from build123d import *

# Parameters (mm, degrees)
SKETCH1_W               = 28
SKETCH1_H               = 55
SKETCH1_R               = 1.25
BOSS_EXTRUDE1_DEPTH     = 6
SKETCH2_W               = 6
SKETCH2_H               = 55
BOSS_EXTRUDE2_DEPTH     = 14.5
SKETCH3_W               = 6
SKETCH3_H               = 55
BOSS_EXTRUDE3_DEPTH     = 48
SKETCH4_R               = 3
SKETCH4_R_2             = 11
CUT_EXTRUDE1_DEPTH      = 48
FILLET4_R               = 2
SKETCH5_W               = 21
SKETCH5_H               = 42
CUT_EXTRUDE2_DEPTH      = 10
FILLET5_R               = 2
ESQUISSE2_R             = 5
BOSS_EXTRU_3_DEPTH      = 41
ESQUISSE3_R             = 1.75
ENL_V_MAT_EXTRU_1_DEPTH = 105.928547117
ESQUISSE4_W             = 76
ESQUISSE4_H             = 20.5
BOSS_EXTRU_4_DEPTH      = 14
ESQUISSE5_W             = 76
ESQUISSE5_H             = 20.5
BOSS_EXTRU_5_DEPTH      = 14
ESQUISSE7_R             = 5
BOSS_EXTRU_8_DEPTH      = 26.5
ESQUISSE10_R            = 1.75
ENL_V_MAT_EXTRU_2_DEPTH = 113.898184219
ENL_V_MAT_EXTRU_3_DEPTH = 4.1
ENL_V_MAT_EXTRU_4_DEPTH = 4.1


with BuildPart() as part:
    # Sketch1 → Boss-Extrude1 (new body)
    with BuildSketch(Plane.XY):
        with Locations((14, 27.5)):
            Rectangle(SKETCH1_W, SKETCH1_H)
        with Locations((5, 52)):
            Circle(SKETCH1_R, mode=Mode.SUBTRACT)
        with Locations((15, 52)):
            Circle(SKETCH1_R, mode=Mode.SUBTRACT)
        with Locations((5, 3)):
            Circle(SKETCH1_R, mode=Mode.SUBTRACT)
        with Locations((15, 3)):
            Circle(SKETCH1_R, mode=Mode.SUBTRACT)
    extrude(amount=BOSS_EXTRUDE1_DEPTH)

    # Sketch2 → Boss-Extrude2 (add)
    with BuildSketch(Plane.XY.offset(6)):
        with Locations((25, 27.5)):
            Rectangle(SKETCH2_W, SKETCH2_H)
    extrude(amount=BOSS_EXTRUDE2_DEPTH)

    # Sketch3 → Boss-Extrude3 (add)
    with BuildSketch(Plane(origin=(28, 0, 0), x_dir=(0, 0, -1), z_dir=(1, 0, 0))):
        with Locations((-17.5, 27.5)):
            Rectangle(SKETCH3_W, SKETCH3_H)
    extrude(amount=BOSS_EXTRUDE3_DEPTH)

    # Sketch4 → Cut-Extrude1 (cut)
    with BuildSketch(Plane.XY.offset(20.5)):
        with Locations((61.416247904, 27.5)):
            Circle(SKETCH4_R)
        with Locations((34.041247904, 11.695036381)):
            Circle(SKETCH4_R)
        with Locations((34.041247904, 43.304963619)):
            Circle(SKETCH4_R)
        with Locations((43.166247904, 27.5)):
            Circle(SKETCH4_R_2)
    extrude(amount=-CUT_EXTRUDE1_DEPTH, mode=Mode.SUBTRACT)

    # Fillet4
    fillet4_edges = [part.edges().sort_by_distance(p)[0] for p in [
        (22, 27.5, 20.5),
        (0, 27.5, 6),
        (0, 27.5, 0),
        (76, 27.5, 14.5),
        (28, 27.5, 14.5),
        (28, 27.5, 0),
        (76, 27.5, 20.5),
    ]]
    fillet(fillet4_edges, radius=FILLET4_R)

    # Sketch5 → Cut-Extrude2 (cut)
    with BuildSketch(Plane.XY.offset(6)):
        with Locations((10.5, 27.5)):
            Rectangle(SKETCH5_W, SKETCH5_H)
    extrude(amount=-CUT_EXTRUDE2_DEPTH, mode=Mode.SUBTRACT)

    # Fillet5
    # the kernel refuses this fillet: 2 mm, written as the material it adds along each edge
    with BuildSketch(Plane(origin=(22, 55, 6), x_dir=(-1, 0, 0), z_dir=(0, -1, 0))) as fillet5_piece_1_section:
        with BuildLine():
            CenterArc((FILLET5_R, -FILLET5_R), FILLET5_R, 90, 90)
            Line((0, -FILLET5_R), (0, 0))
            Line((0, 0), (FILLET5_R, 0))
        make_face()
    fillet5_piece_1 = extrude(amount=55, mode=Mode.PRIVATE)
    fillet5_piece_1 = split(fillet5_piece_1, bisect_by=Plane(origin=(21, 51.75, 6.048016763), z_dir=(-1, 0, 0)), keep=Keep.TOP, mode=Mode.PRIVATE)
    fillet5_piece_1 = split(fillet5_piece_1, bisect_by=Plane(origin=(20.673498431, 48.5, 6.048016763), z_dir=(0, 1, 0)), keep=Keep.TOP, mode=Mode.PRIVATE)
    add(fillet5_piece_1)
    with BuildSketch(Plane(origin=(22, 55, 6), x_dir=(-1, 0, 0), z_dir=(0, -1, 0))) as fillet5_piece_2_section:
        with BuildLine():
            CenterArc((FILLET5_R, -FILLET5_R), FILLET5_R, 90, 90)
            Line((0, -FILLET5_R), (0, 0))
            Line((0, 0), (FILLET5_R, 0))
        make_face()
    fillet5_piece_2 = extrude(amount=55, mode=Mode.PRIVATE)
    fillet5_piece_2 = split(fillet5_piece_2, bisect_by=Plane(origin=(21, 51.75, 6.51024012), z_dir=(1, 0, 0)), keep=Keep.TOP, mode=Mode.PRIVATE)
    fillet5_piece_2 = split(fillet5_piece_2, bisect_by=Plane(origin=(21.671216471, 48.5, 6.51024012), z_dir=(0, 1, 0)), keep=Keep.TOP, mode=Mode.PRIVATE)
    add(fillet5_piece_2)
    with BuildSketch(Plane(origin=(22, 55, 6), x_dir=(-1, 0, 0), z_dir=(0, -1, 0))) as fillet5_piece_3_section:
        with BuildLine():
            CenterArc((FILLET5_R, -FILLET5_R), FILLET5_R, 90, 90)
            Line((0, -FILLET5_R), (0, 0))
            Line((0, 0), (FILLET5_R, 0))
        make_face()
    fillet5_piece_3 = extrude(amount=55, mode=Mode.PRIVATE)
    fillet5_piece_3 = split(fillet5_piece_3, bisect_by=Plane(origin=(21.671216471, 6.5, 6.51024012), z_dir=(0, 1, 0)), keep=Keep.TOP, mode=Mode.PRIVATE)
    fillet5_piece_3 = split(fillet5_piece_3, bisect_by=Plane(origin=(21, 27.5, 6.51024012), z_dir=(1, 0, 0)), keep=Keep.TOP, mode=Mode.PRIVATE)
    fillet5_piece_3 = split(fillet5_piece_3, bisect_by=Plane(origin=(21.671216471, 48.5, 6.51024012), z_dir=(0, -1, 0)), keep=Keep.TOP, mode=Mode.PRIVATE)
    add(fillet5_piece_3)
    with BuildSketch(Plane(origin=(22, 55, 6), x_dir=(-1, 0, 0), z_dir=(0, -1, 0))) as fillet5_piece_4_section:
        with BuildLine():
            CenterArc((FILLET5_R, -FILLET5_R), FILLET5_R, 90, 90)
            Line((0, -FILLET5_R), (0, 0))
            Line((0, 0), (FILLET5_R, 0))
        make_face()
    fillet5_piece_4 = extrude(amount=55, mode=Mode.PRIVATE)
    fillet5_piece_4 = split(fillet5_piece_4, bisect_by=Plane(origin=(20.673498431, 6.5, 6.048016763), z_dir=(0, -1, 0)), keep=Keep.TOP, mode=Mode.PRIVATE)
    fillet5_piece_4 = split(fillet5_piece_4, bisect_by=Plane(origin=(21, 3.25, 6.048016763), z_dir=(-1, 0, 0)), keep=Keep.TOP, mode=Mode.PRIVATE)
    add(fillet5_piece_4)
    with BuildSketch(Plane(origin=(22, 55, 6), x_dir=(-1, 0, 0), z_dir=(0, -1, 0))) as fillet5_piece_5_section:
        with BuildLine():
            CenterArc((FILLET5_R, -FILLET5_R), FILLET5_R, 90, 90)
            Line((0, -FILLET5_R), (0, 0))
            Line((0, 0), (FILLET5_R, 0))
        make_face()
    fillet5_piece_5 = extrude(amount=55, mode=Mode.PRIVATE)
    fillet5_piece_5 = split(fillet5_piece_5, bisect_by=Plane(origin=(21.671216471, 6.5, 6.51024012), z_dir=(0, -1, 0)), keep=Keep.TOP, mode=Mode.PRIVATE)
    fillet5_piece_5 = split(fillet5_piece_5, bisect_by=Plane(origin=(21, 3.25, 6.51024012), z_dir=(1, 0, 0)), keep=Keep.TOP, mode=Mode.PRIVATE)
    add(fillet5_piece_5)

    # Esquisse2 → Boss.-Extru.3 (add)
    with BuildSketch(Plane(origin=(0, 0, 14.5), x_dir=(-1, 0, 0), z_dir=(0, 0, -1))):
        with Locations(Location((-69, 47.5, 0), (0, 0, 180))):
            Circle(ESQUISSE2_R)
        with Locations(Location((-69, 7.5, 0), (0, 0, 180))):
            Circle(ESQUISSE2_R)
    extrude(amount=BOSS_EXTRU_3_DEPTH)

    # Esquisse3 → Enlèv. mat.-Extru.1 (cut, through all)
    with BuildSketch(Plane(origin=(0, 0, -26.5), x_dir=(-1, 0, 0), z_dir=(0, 0, -1))):
        with Locations(Location((-69, 7.5, 0), (0, 0, 90))):
            Circle(ESQUISSE3_R)
        with Locations(Location((-69, 47.5, 0), (0, 0, 90))):
            Circle(ESQUISSE3_R)
    extrude(amount=-ENL_V_MAT_EXTRU_1_DEPTH, mode=Mode.SUBTRACT)

    # Esquisse4 → Boss.-Extru.4 (add)
    with BuildSketch(Plane(origin=(0, 55, 0), x_dir=(1, 0, 0), z_dir=(0, 1, 0))):
        with Locations((38, -10.25)):
            Rectangle(ESQUISSE4_W, ESQUISSE4_H)
    extrude(amount=BOSS_EXTRU_4_DEPTH)

    # Esquisse5 → Boss.-Extru.5 (add)
    with BuildSketch(Plane.XZ):
        with Locations((38, 10.25)):
            Rectangle(ESQUISSE5_W, ESQUISSE5_H)
    extrude(amount=BOSS_EXTRU_5_DEPTH)

    # Esquisse7 → Boss.-Extru.8 (add)
    with BuildSketch(Plane(origin=(0, 0, 0), x_dir=(-1, 0, 0), z_dir=(0, 0, -1))):
        with Locations((-7.5, -7.5)):
            Circle(ESQUISSE7_R)
        with Locations((-7.5, 62.5)):
            Circle(ESQUISSE7_R)
    extrude(amount=BOSS_EXTRU_8_DEPTH)

    # Esquisse10 → Enlèv. mat.-Extru.2 (cut, through all)
    with BuildSketch(Plane(origin=(0, 0, -26.5), x_dir=(-1, 0, 0), z_dir=(0, 0, -1))):
        with Locations((-7.5, 62.5)):
            Circle(ESQUISSE10_R)
        with Locations((-7.5, -7.5)):
            Circle(ESQUISSE10_R)
    extrude(amount=-ENL_V_MAT_EXTRU_2_DEPTH, mode=Mode.SUBTRACT)

    # Esquisse11 → Enlèv. mat.-Extru.3 (cut)
    with BuildSketch(Plane(origin=(0, 0, -26.5), x_dir=(-1, 0, 0), z_dir=(0, 0, -1))):
        Polygon((-9.145448267, -4.65), (-10.790896534, -7.5), (-9.145448267, -10.35), (-5.854551733, -10.35), (-4.209103466, -7.5), (-5.854551733, -4.65), align=None)
    extrude(amount=-ENL_V_MAT_EXTRU_3_DEPTH, mode=Mode.SUBTRACT)

    # Esquisse12 → Enlèv. mat.-Extru.4 (cut)
    with BuildSketch(Plane(origin=(0, 0, -26.5), x_dir=(-1, 0, 0), z_dir=(0, 0, -1))):
        Polygon((-9.145448267, 65.35), (-10.790896534, 62.5), (-9.145448267, 59.65), (-5.854551733, 59.65), (-4.209103466, 62.5), (-5.854551733, 65.35), align=None)
        Polygon((-70.645448267, 50.35), (-72.290896534, 47.5), (-70.645448267, 44.65), (-67.354551733, 44.65), (-65.709103466, 47.5), (-67.354551733, 50.35), align=None)
        Polygon((-70.645448267, 10.35), (-72.290896534, 7.5), (-70.645448267, 4.65), (-67.354551733, 4.65), (-65.709103466, 7.5), (-67.354551733, 10.35), align=None)
    extrude(amount=-ENL_V_MAT_EXTRU_4_DEPTH, mode=Mode.SUBTRACT)


solid = part.part
Could you check a few things on this model? Use its own coordinates, in mm. A direction names the side the tool comes from. Round coordinates to 2 decimals unless told otherwise and drop trailing zeros. Write each loop counter-clockwise with the first axis right and the second up, starting at its lowest first coordinate (ties: lowest second). Pieces come first, ordered by that corner, then holes. Notation, with made-up numbers: (32.25, -18.5) - (65.25, -18.5) arc R25 cw to (65.25, 20.5) - close; hole circle Ø11 at (-5, -1.5). An arc over 180 degrees is marked (long way). Use a Markdown table: item, result.
Q1. I want a section at D-D (x = 69). Count the separate pieces of the cut face and the enclosed holes in it, plus the area to 3 significant figures.
Output values:
| item | result |
|---|---|
| separate pieces | 3 |
| enclosed holes | 0 |
| area | 1,380 mm2 |
Q2. Please list where these lines run through material, in increasing order: L1, parallel to Y at x = 59, z = 9; L2, parallel to X at y = 7, z = 10.5; L3, parallel to Y at x = 69, z = 8.
Output values:
| item | result |
|---|---|
| L1 | -14 to 0, 55 to 69 |
| L2 | 22 to 28, 64.03 to 67.32, 70.68 to 73.97 |
| L3 | -14 to 0, 2.5 to 5.75, 9.25 to 12.5, 42.5 to 45.75, 49.25 to 52.5, 55 to 69 |
Q3. I want a section at B-B (y = 27.5). List the corners of the cut face in (x, z) for me, plus the area to 3 significant figures.
Output values:
| item | result |
|---|---|
| outline | (21, 0) - (26, 0) arc R2 ccw to (28, 2) - (28, 12.5) arc R2 cw to (30, 14.5) - (32.17, 14.5) - (32.17, 20.5) - (24, 20.5) arc R2 ccw to (22, 18.5) - (22, 8) arc R2 cw to (21, 6.27) - close; (54.17, 14.5) - (58.42, 14.5) - (58.42, 20.5) - (54.17, 20.5) - close; (64.42, 14.5) - (74, 14.5) arc R2 ccw to (76, 16.5) - (76, 18.5) arc R2 ccw to (74, 20.5) - (64.42, 20.5) - close |
| area | 247 mm2 |
Q4. I want a section at A-A (z = -9). List the corners of the cut face in (x, y) for me, plus the area to 3 significant figures.
Output values:
| item | result |
|---|---|
| outline | circle Ø10 at (7.5, -7.5); circle Ø10 at (7.5, 62.5); circle Ø10 at (69, 7.5); circle Ø10 at (69, 47.5); hole circle Ø3.5 at (7.5, -7.5); hole circle Ø3.5 at (7.5, 62.5); hole circle Ø3.5 at (69, 7.5); hole circle Ø3.5 at (69, 47.5) |
| area | 276 mm2 |
Q5. I want a section at C-C (x = 55.5). List the corners of the cut face in (y, z) for me.
Output values:
| item | result |
|---|---|
| outline | (-14, 0) - (0, 0) - (0, 14.5) - (55, 14.5) - (55, 0) - (69, 0) - (69, 20.5) - (-14, 20.5) - close |
Q6. For pin 1 (5 mm diameter, centred on x = 14, z = -17.5, fed in from -Y); pin 2 (1.7 mm diameter, centred on x = 8.5, y = -6.5, fed in from -Z); pin 3 (2.5 mm diameter, centred on x = 6.5, z = -24, fed in from -Y); pin 4 (2 mm diameter, centred on x = 7.5, y = -7.5, fed in from -Z), each with a flat end and sliding along its axis, tell me the tip position at first contact or that it passes through.
Output values:
| item | result |
|---|---|
| pin 1 | y = -10.5 |
| pin 2 | z = -22.4 |
| pin 3 | y = -12.5 |
| pin 4 | through |
Q7. Thinking about a two-plate mould opening in Y: for faces 1 (the flat face through (5, -10, -26.5)), 2 (the flat face through (0.4, 0, 0.5)), which applies, released by +Y, released by -Y, zero draft, split by the parting line, or undercut?
Output values:
| item | result |
|---|---|
| face 1 | zero draft |
| face 2 | undercut |
Q8. For faces 3 (the cylindrical face through (73.619, 9.415, -5.713)), 4 (the flat face through (22, 27, 13)), 5 (the flat face through (11, 48.5, 3)), which set-ups out of +Z, -Z, +X, -X, +Y, -Y let a thin tool reach every point of the face, with its end or its side?
Output values:
| item | result |
|---|---|
| face 3 | -Z |
| face 4 | +Z, -X |
| face 5 | +Z, -Z, -X |
